from build123d import *

# Parameters (mm, degrees)
SKETCH1_R           = 15
SKETCH1_R_2         = 1.5
BOSS_EXTRUDE1_DEPTH = 3.175
CUT_EXTRUDE1_DEPTH  = 3.175


with BuildPart() as part:
    # Sketch1 → Boss-Extrude1 (new body)
    with BuildSketch(Plane(origin=(0, 0, 0), x_dir=(1, 0, 0), z_dir=(0, 1, 0))):
        with Locations(Location((0, 0, 0), (0, 0, 270))):
            Circle(SKETCH1_R)
        with Locations(Location((-8.825381331, 7.093668739, 0), (0, 0, 270))):
            Circle(SKETCH1_R_2, mode=Mode.SUBTRACT)
        with Locations(Location((4.019287066, 10.585500617, 0), (0, 0, 270))):
            Circle(SKETCH1_R_2, mode=Mode.SUBTRACT)
        with Locations(Location((11.309437348, -0.55146957, 0), (0, 0, 270))):
            Circle(SKETCH1_R_2, mode=Mode.SUBTRACT)
        with Locations(Location((2.970329609, -10.926327555, 0), (0, 0, 270))):
            Circle(SKETCH1_R_2, mode=Mode.SUBTRACT)
        with Locations(Location((-9.473672692, -6.201372231, 0), (0, 0, 270))):
            Circle(SKETCH1_R_2, mode=Mode.SUBTRACT)
    extrude(amount=BOSS_EXTRUDE1_DEPTH)

    # Sketch2 → Cut-Extrude1 (cut)
    with BuildSketch(Plane(origin=(0, 3.175, 0), x_dir=(1, 0, 0), z_dir=(0, 1, 0))):
        with BuildLine():
            Line((2.818653923, -1.027224446), (1.934730022, 2.292775554))
            ThreePointArc((1.934730022, 2.292775554), (-2.899010992, -0.771838887), (2.818653923, -1.027224446))
        make_face()
    extrude(amount=-CUT_EXTRUDE1_DEPTH, mode=Mode.SUBTRACT)


solid = part.part
Part model, mm, in its own coordinate system. A direction names the side the tool comes from. Coordinates: 2 decimals unless noted, no trailing zeros. Order: outer loops, then holes, each group sorted by start corner. A loop starts at its lowest first (then second) coordinate and runs counter-clockwise, first axis right, second up. Notation, with made-up numbers: M 84,42 L 135,42 A26 cw 135,81 Z; hole C 72,44 d2. An arc over 180 degrees is marked long. Use a Markdown table: item, result.
(1) Tool access for faces 4 (the flat face through (4, 3.175, 0)), 5 (the flat face through (2.383, 1.61, -0.61)): list every direction of +Z, -Z, +X, -X, +Y, -Y with a clear straight run to the whole face (end or side of a thin tool).
A:
| item | result |
|---|---|
| face 4 | +Z, -Z, +X, -X, +Y |
| face 5 | +Y, -Y |
(2) Pull direction X, two halves, no side cores. Call faces 1 (the cylindrical face through (0.66, 1.565, -14.985)), 2 (the flat face through (4, 0, 0)), 3 (the cylindrical face through (-7.81, 1.57, -8.2)): released by +X, released by -X, zero draft, split by the parting line, or undercut.
A:
| item | result |
|---|---|
| face 1 | split by the parting line |
| face 2 | zero draft |
| face 3 | undercut |
(3) Cut at D-D on y = 0.85. Write the cut outline in (x, z).
A:
| item | result |
|---|---|
| outline | C 0,0 d30; hole C -9.47,6.2 d3; hole C -8.83,-7.09 d3; hole C 2.97,10.93 d3; hole M 1.93,-2.29 L 2.82,1.03 A3 ccw long Z; hole C 4.02,-10.59 d3; hole C 11.31,0.55 d3 |
(4) Cut at C-C on z = -6. Write the cut outline in (x, y) (3 decimals), then the cut area to 3 significant figures.
A:
| item | result |
|---|---|
| outline | M -13.748,0 L -9.852,0 L -9.852,3.175 L -13.748,3.175 Z; M -7.799,0 L 13.748,0 L 13.748,3.175 L -7.799,3.175 Z |
| area | 80.8 mm^2 |
(5) Cut at A-A on x = 0. Write the cut outline in (y, z) (3 decimals), then the cut area to 3 significant figures.
A:
| item | result |
|---|---|
| outline | M 0,-15 L 3.175,-15 L 3.175,-3 L 0,-3 Z; M 0,3 L 3.175,3 L 3.175,15 L 0,15 Z |
| area | 76.2 mm^2 |
(6) Probe L1, parallel to Z at x = -8.25, y = 0.4; L2, parallel to Z at x = 4.75, y = 1.5; L3, parallel to X at y = 2.95, z = 10.5. List the from-to ranges inside material, lowest first.
A:
| item | result |
|---|---|
| L1 | z = -12.53 to -8.48, -5.71 to 5.33, 7.07 to 12.53 |
| L2 | z = -14.23 to -11.9, -9.28 to 14.23 |
| L3 | x = -10.71 to 1.53, 4.41 to 10.71 |
(7) Cut at B-B on z = 0. Write the cut outline in (x, y) (3 decimals).
A:
| item | result |
|---|---|
| outline | M -15,0 L -3,0 L -3,3.175 L -15,3.175 Z; M 2.545,0 L 9.914,0 L 9.914,3.175 L 2.545,3.175 Z; M 12.704,0 L 15,0 L 15,3.175 L 12.704,3.175 Z |
